Read the model definition and answer for the solid it produces. Units are mm, in the model's axes. A direction names the side the tool comes from. Coordinates: 2 decimals unless noted, no trailing zeros. Write each loop counter-clockwise with the first axis right and the second up, starting at its lowest first coordinate (ties: lowest second). Pieces come first, ordered by that corner, then holes. Notation, with made-up numbers: (70, 6) - (115, 6) arc R13 cw to (115, 15) - close; hole circle Ø8 at (2.5, -31). An arc over 180 degrees is marked (long way). Return JSON: item names as keys, results as strings.
```python
from build123d import *

# Parameters (mm, degrees)
F1_DEPTH = 304.8
F2_R     = 9.525
F3_DEPTH = 25.4
F5_DEPTH = 25.4


with BuildPart() as f1:
    # F0 (on Front) → F1 (new body, symmetric)
    with BuildSketch(Plane.XZ):
        with BuildLine():
            ThreePointArc((12.7, 23.876), (12.253631, 24.953631), (11.176, 25.4))
            Line((11.176, 25.4), (-11.176, 25.4))
            ThreePointArc((-11.176, 25.4), (-12.253631, 24.953631), (-12.7, 23.876))
            Line((-12.7, 23.876), (-12.7, -23.876))
            ThreePointArc((-12.7, -23.876), (-12.253631, -24.953631), (-11.176, -25.4))
            Line((-11.176, -25.4), (11.176, -25.4))
            ThreePointArc((11.176, -25.4), (12.253631, -24.953631), (12.7, -23.876))
            Line((12.7, -23.876), (12.7, 23.876))
        make_face()
        with BuildLine():
            Line((-8.128, 22.352), (8.128, 22.352))
            ThreePointArc((8.128, 22.352), (9.205631, 21.905631), (9.652, 20.828))
            Line((9.652, 20.828), (9.652, -20.828))
            ThreePointArc((9.652, -20.828), (9.205631, -21.905631), (8.128, -22.352))
            Line((8.128, -22.352), (-8.128, -22.352))
            ThreePointArc((-8.128, -22.352), (-9.205631, -21.905631), (-9.652, -20.828))
            Line((-9.652, -20.828), (-9.652, 20.828))
            ThreePointArc((-9.652, 20.828), (-9.205631, 21.905631), (-8.128, 22.352))
        make_face(mode=Mode.SUBTRACT)
    extrude(amount=F1_DEPTH, both=True)

    # F2 (on face) → F3 (cut)
    with BuildSketch(Plane.YZ.offset(12.7)):
        with Locations((-279.4, 0)):
            Circle(F2_R)
        with Locations((279.4, 0)):
            Circle(F2_R)
    extrude(amount=-F3_DEPTH, mode=Mode.SUBTRACT)

    # F4 (on face) → F5 (cut)
    with BuildSketch(Plane.YZ.offset(12.7)):
        with BuildLine():
            ThreePointArc((-279.4, -25.4), (-304.8, 0), (-279.4, 25.4))
            Line((-279.4, 25.4), (-279.4, 43.210469))
            Line((-279.4, 43.210469), (-315.057784, 43.210469))
            Line((-315.057784, 43.210469), (-315.057784, -40.735509))
            Line((-315.057784, -40.735509), (-279.4, -40.735509))
            Line((-279.4, -40.735509), (-279.4, -25.4))
        make_face()
        with BuildLine():
            Line((315.057784, -40.735509), (315.057784, 43.210469))
            Line((315.057784, 43.210469), (279.4, 43.210469))
            Line((279.4, 43.210469), (279.4, 25.4))
            ThreePointArc((279.4, 25.4), (304.8, 0), (279.4, -25.4))
            Line((279.4, -25.4), (279.4, -40.735509))
            Line((279.4, -40.735509), (315.057784, -40.735509))
        make_face()
    extrude(amount=-F5_DEPTH, mode=Mode.SUBTRACT)


solid = f1.part
```
(1) A cutting plane is placed at C-C (y = -120). Determine the outline of the cut face in (x, z), and give its area (3 significant figures).
Answer:
{"outline": "(-12.7, -23.88) arc R1.52 ccw to (-11.18, -25.4) - (11.18, -25.4) arc R1.52 ccw to (12.7, -23.88) - (12.7, 23.88) arc R1.52 ccw to (11.18, 25.4) - (-11.18, 25.4) arc R1.52 ccw to (-12.7, 23.88) - close; hole (-9.65, -20.83) arc R1.52 ccw to (-8.13, -22.35) - (8.13, -22.35) arc R1.52 ccw to (9.65, -20.83) - (9.65, 20.83) arc R1.52 ccw to (8.13, 22.35) - (-8.13, 22.35) arc R1.52 ccw to (-9.65, 20.83) - close", "area": "427 mm²"}
(2) Determine the mould class of faces 3 (the face through (-12.7, -4, 0)), 4 (the face through (11.197, -270.315, 2.861)), 5 (the face through (9.652, -4, 0)) for opening direction X: +X half, -X half, draft (parallel to the pull), parting line (faces both ways), or undercut.
Answer:
{"face 3": "-X half", "face 4": "draft", "face 5": "undercut"}
(3) Which of the six approach directions +Z, -Z, +X, -X, +Y, -Y give full straight-line access (tool end or side, diameter ignored) to faces 1 (the face through (11.467, -304.794, -0.559)), 2 (the face through (0, -4, -22.352))?
Answer:
{"face 1": "+X, -X, -Y", "face 2": "+Y, -Y"}
(4) Straight lines are drawn through the part: line 1 (X direction, y = -50.5, z = -18.5); line 2 (Z direction, x = -1.25, y = -210). For each, find the intervals that lie inside material, in ascending order. Write a range as from..to.
Answer:
{"line 1": "-12.7..-9.65, 9.65..12.7", "line 2": "-25.4..-22.35, 22.35..25.4"}
(5) A flat-ended cylindrical pin translates along its axis: P1, Ø8, axis at x = 8.5, z = 12.5, coming from the +Y side. Find the tip coordinate at first contact, or state that the pin passes through.
Answer:
{"P1": "y = 303.27"}
(6) A cutting plane is placed at B-B (z = 0). Determine the outline of the cut face in (x, y) (3 decimals), and give its area (3 significant figures).
Answer:
{"outline": "(-12.7, -304.8) - (-9.652, -304.8) - (-9.652, -288.925) - (-12.7, -288.925) - close; (-12.7, -269.875) - (-9.652, -269.875) - (-9.652, 269.875) - (-12.7, 269.875) - close; (-12.7, 288.925) - (-9.652, 288.925) - (-9.652, 304.8) - (-12.7, 304.8) - close; (9.652, -304.8) - (12.7, -304.8) - (12.7, -288.925) - (9.652, -288.925) - close; (9.652, -269.875) - (12.7, -269.875) - (12.7, 269.875) - (9.652, 269.875) - close; (9.652, 288.925) - (12.7, 288.925) - (12.7, 304.8) - (9.652, 304.8) - close", "area": "3,480 mm²"}
(7) A cutting plane is placed at A-A (x = -0.5). Determine the outline of the cut face in (y, z).
Answer:
{"outline": "(-291.46, -22.35) arc R25.4 ccw to (-279.4, -25.4) - (279.4, -25.4) arc R25.4 ccw to (291.46, -22.35) - close; (-291.46, 22.35) - (291.46, 22.35) arc R25.4 ccw to (279.4, 25.4) - (-279.4, 25.4) arc R25.4 ccw to start"}
